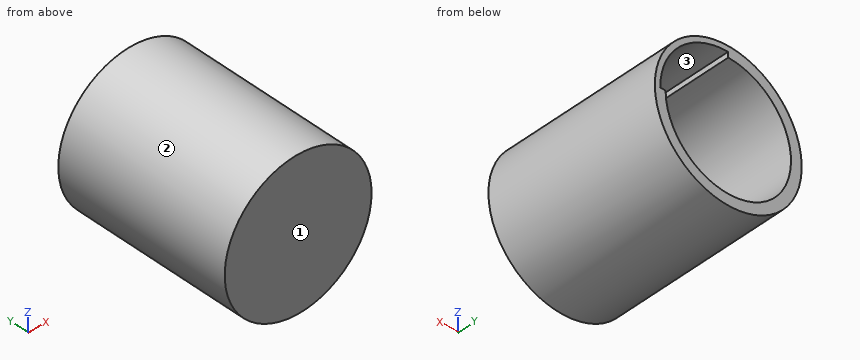
Autodesk Fusion 360 part; units mm, degrees
sketch "Sketch1" plane through (0, 0, 0) normal (0, 1, 0) x (1, 0, 0)
  circle A0 centre (0, 0) radius 41
  circle A1 centre (0, 0) radius 35
  line L0 (0.0406, -35) -> (0.0406, -38)
  line L1 (35, 0.0176) -> (38, 0.0176)
  arc A2 (0.0406, -38) -> (38, 0.0176) centre (0, 0) ccw
  dimension "d1" = 82
  dimension "d2" = 70
extrude "Extrude1" add sketch "Sketch1" along normal blind 100
extrude "Extrude2" add sketch "Sketch1" along normal blind 6 contours A1
extrude "Extrude3" add sketch "Sketch1" along normal blind 6 contours A1 L0 L1 A2
sketch "Sketch2" plane through (0, 6, 0) normal (0, 1, 0) x (-1, 0, 0)
  line L0 (-0.0406, 35) -> (-0.0406, 38)
  arc A0 (-0.0406, 38) -> (-38, -0.0176) centre (0, 0) ccw
  line L1 (-38, -0.0176) -> (-35, -0.0176)
  circle A1 centre (0, 0) radius 26
  arc A2 (-35, -0.0176) -> (-0.0406, 35) centre (0, 0) ccw
  dimension "d10" = 52
extrude "Extrude4" cut sketch "Sketch2" against normal blind 4 contours A1
Part model, mm, in its own coordinate system. Face numbers are marked on the shaded views. Give positions to 0.01 mm unless a question says otherwise; leave off trailing zeros. Order: outer loops, then holes, each group sorted by start corner. A loop starts at its lowest first (then second) coordinate and runs counter-clockwise, first axis right, second up. Notation, with made-up numbers: (46, 68) -> (81, 68) arc R31 cw to (81, 106) -> close; hole circle Ø4 at (-31, 69.25). An arc over 180 degrees is marked (long way). Use one line per item in the form item = value.
(1) Drill centre lines: line 1 (Z direction, x = -1, y = 9.5); line 2 (X direction, y = 10, z = 1); line 3 (X direction, y = 61, z = -32). Where is each one in solid material? Low to high. Write a range as from..to.
Solution:
line_1 = -40.99..-34.99, 34.99..40.99
line_2 = -40.99..-34.99, 37.99..40.99
line_3 = -25.63..-14.18, 14.18..25.63
(2) Saw through at A-A (z = 23.5). Write the cut outline in (x, y).
Solution:
outline = (-33.6, 0) -> (33.6, 0) -> (33.6, 100) -> (29.86, 100) -> (29.86, 6) -> (11.12, 6) -> (11.12, 2) -> (-11.12, 2) -> (-11.12, 6) -> (-25.94, 6) -> (-25.94, 100) -> (-33.6, 100) -> close
(3) Saw through at C-C (y = 22). Write the cut outline in (x, z).
Solution:
outline = circle Ø82 at (0, 0); hole (0.04, 35) arc R35 ccw (long way) to (35, -0.02) -> (38, -0.02) arc R38 ccw to (0.04, 38) -> close
(4) Flat gauge pins, fed straight in: P1, Ø1, axis at y = 80.5, z = 31.5, coming from the +X side; P2, Ø12, axis at y = 16, z = 20, coming from the +X side; P3, Ø6, axis at x = -22, y = 36, coming from the +Z side. Where does each tip first touch, or does it go through?
Solution:
P1 = 26.83
P2 = 38.54
P3 = 36.33
(5) Saw through at B-B (x = 11). Write the cut outline in (y, z), then the cut area to 3 significant figures.
Solution:
outline = (0, -39.5) -> (100, -39.5) -> (100, -33.23) -> (6, -33.23) -> (6, -23.56) -> (2, -23.56) -> (2, 23.56) -> (6, 23.56) -> (6, 36.37) -> (100, 36.37) -> (100, 39.5) -> (0, 39.5) -> close
area = 1,170 mm²
(6) Pull direction X, two halves, no side cores. Call the marked faces 1, 2 and 3: +X half, -X half, draft (parallel to the pull), parting line (faces both ways), or undercut.
Solution:
face_1 = draft
face_2 = parting line
face_3 = undercut
